from build123d import *

# Parameters (mm, degrees)
SKETCH1_R           = 2.25
BOSS_EXTRUDE1_DEPTH = 25.4
SKETCH2_R           = 2.25
SKETCH2_W           = 12.7
SKETCH2_H           = 12.7
CUT_EXTRUDE1_DEPTH  = 12.7
FILLET1_R           = 6.35
FILLET2_R           = 6.35


with BuildPart() as part:
    # Sketch1 → Boss-Extrude1 (new body)
    with BuildSketch(Plane(origin=(0, 0, 0), x_dir=(1, 0, 0), z_dir=(0, 1, 0))):
        Polygon((158.75, 44.45), (158.75, 31.75), (6.35, 31.75), (6.35, -6.35), (-6.35, -6.35), (-6.35, 31.75), (-19.05, 31.75), (-19.05, 44.45), align=None)
        with Locations(Location((0, 38.1, 0), (0, 0, 270))):
            Circle(SKETCH1_R, mode=Mode.SUBTRACT)
        with Locations(Location((152.4, 38.1, 0), (0, 0, 270))):
            Circle(SKETCH1_R, mode=Mode.SUBTRACT)
        with Locations(Location((139.7, 38.1, 0), (0, 0, 270))):
            Circle(SKETCH1_R, mode=Mode.SUBTRACT)
        with Locations(Location((0, 25.4, 0), (0, 0, 270))):
            Circle(SKETCH1_R, mode=Mode.SUBTRACT)
        with Locations(Location((0, 12.7, 0), (0, 0, 270))):
            Circle(SKETCH1_R, mode=Mode.SUBTRACT)
        with Locations(Location((0, 0, 0), (0, 0, 270))):
            Circle(SKETCH1_R, mode=Mode.SUBTRACT)
    extrude(amount=BOSS_EXTRUDE1_DEPTH)

    # Sketch2 → Cut-Extrude1 (cut)
    with BuildSketch(Plane.XY.offset(-31.75)):
        with Locations((-12.7, 19.05)):
            Circle(SKETCH2_R)
        with Locations((-12.7, 6.35)):
            Rectangle(SKETCH2_W, SKETCH2_H)
    extrude(amount=-CUT_EXTRUDE1_DEPTH, mode=Mode.SUBTRACT)

    # Fillet1
    fillet1_edges = [part.edges().sort_by_distance(p)[0] for p in [
        (158.75, 12.7, -44.45),
        (158.75, 12.7, -31.75),
        (6.35, 12.7, 6.35),
        (-6.35, 12.7, 6.35),
        (-6.35, 6.35, -44.45),
        (6.35, 12.7, -31.75),
        (-19.05, 12.7, -38.1),
        (-19.05, 25.4, -38.1),
    ]]
    fillet(fillet1_edges, radius=FILLET1_R - 0.0001)  # a hair under: the kernel refuses the full size

    # Fillet2
    fillet2_edges = [part.edges().sort_by_distance(p)[0] for p in [
        (-4.49015735, 12.7, -42.59015735),
        (-6.35, 12.7, -34.92505),
    ]]
    fillet(fillet2_edges, radius=FILLET2_R)


solid = part.part
Here's how the part is built. I have some questions about the finished solid (model axes, mm). A direction names the side the tool comes from. Round coordinates to 2 decimals unless told otherwise and drop trailing zeros. Loops run counter-clockwise (first coordinate to the right, second up) from the corner with the lowest first, then second, coordinate; pieces in that order, holes last. Notation, with made-up numbers: M -39.5,73.5 L 1.5,73.5 A29 cw 1.5,102.5 Z; hole C 42.5,21 d3. An arc over 180 degrees is marked long. Write each question's results on one line, items separated by ' | '. Start each with the question number.
(1) I want a section at C-C (y = 4). State how many separate pieces and enclosed holes the cut face has, then the cut area to 3 significant figures.
(2) Will these pins go through, and if not, where does the flat tip stop? P1, Ø12, axis at y = 5, z = -8, coming from the +X side; P2, Ø3.5, axis at x = 0, z = -12.7, coming from the -Y side; P3, Ø12.5, axis at y = 9.5, z = -24.5, coming from the -X side; P4, Ø5, axis at x = -12.7, y = 19.05, coming from the +Z side.
(3) I want a section at D-D (z = -6). Please give me the cut outline in (x, y).
(4) I want a section at B-B (z = -12.7). Please give me the cut outline in (x, y).
(5) I want a section at A-A (x = 139.7). Please give me the cut outline in (y, z), then the cut area to 3 significant figures.
(6) On a 3-axis mill with a long thin cutter (end or side, diameter ignored), from which of +Z, -Z, +X, -X, +Y, -Y can I reach the whole of each face in a straight line? I mean faces 1 (the cylindrical face through (-4.54, 3.22, -42.54)), 2 (the flat face through (64, 0, -34)). Say none if no direction works.
(7) Thinking about a two-plate mould opening in Z: for faces 3 (the cylindrical face through (0.099, 12.522, -27.648)), 4 (the cylindrical face through (150.404, 12.522, -37.062)), 5 (the flat face through (84, 13, -31.75)), 6 (the flat face through (6.35, 13, -13)), which applies, pulls with the +Z half, pulls with the -Z half, needs draft (parallel to the pull), parting line crosses it, or undercut?
(8) If I drill on probe 1 along Z at (x, y) = (139.5, 3); probe 2 along X at (y, z) = (7.25, -12.7); probe 3 along Y at (x, z) = (-12.7, -39.5), over which ranges is the centre line in solid material (lowest first)? Write a range as from..to.
Solved:
1) separate pieces: 1 | enclosed holes: 6 | area: 2,450 mm²
2) P1: stops at x = 6.35 | P2: passes through | P3: stops at x = -6.35 | P4: stops at z = -31.75
3) outline: M -6.35,0 L 6.35,0 L 6.35,25.4 L -6.35,25.4 Z
4) outline: M -6.35,0 L -2.25,0 L -2.25,25.4 L -6.35,25.4 Z; M 2.25,0 L 6.35,0 L 6.35,25.4 L 2.25,25.4 Z
5) outline: M 0,-44.45 L 25.4,-44.45 L 25.4,-40.35 L 0,-40.35 Z; M 0,-35.85 L 25.4,-35.85 L 25.4,-31.75 L 0,-31.75 Z | area: 208 mm²
6) face 1: -Z, -X, -Y | face 2: +Z, -Z, +X, -X, -Y
7) face 3: undercut | face 4: undercut | face 5: pulls with the +Z half | face 6: needs draft
8) probe 1: z = -44.45..-40.34, -35.86..-31.75 | probe 2: x = -6.35..-2.25, 2.25..6.35 | probe 3: y = 12.7..16.8, 21.3..25.4
